```python
from build123d import *

# Parameters (mm, degrees)
SKETCH2_R           = 37.5
BOSS_EXTRUDE1_DEPTH = 6.75
SKETCH3_R           = 7.95
BOSS_EXTRUDE2_DEPTH = 150
BOSS_EXTRUDE3_DEPTH = 27


with BuildPart() as part:
    # Sketch2 → Boss-Extrude1 (new body, symmetric)
    with BuildSketch(Plane(origin=(0, 0, 0), x_dir=(1, 0, 0), z_dir=(0, 1, 0))):
        Polygon((-107, -100), (-40, -160), (40, -160), (107, -100), (107, 100), (-107, 100), align=None)
        Circle(SKETCH2_R, mode=Mode.SUBTRACT)
    extrude(amount=BOSS_EXTRUDE1_DEPTH, both=True)

    # Sketch3 → Boss-Extrude2 (add)
    with BuildSketch(Plane.XZ.offset(6.75)):
        with Locations((26.625, 147.55)):
            Circle(SKETCH3_R)
        with Locations((-26.625, 147.55)):
            Circle(SKETCH3_R)
    extrude(amount=BOSS_EXTRUDE2_DEPTH)

    # Sketch4 → Boss-Extrude3 (add)
    with BuildSketch(Plane.XZ.offset(156.75)):
        with BuildLine():
            Line((-45, 72), (-45, 160))
            Line((-45, 160), (45, 160))
            Line((45, 160), (45, 72))
            ThreePointArc((45, 72), (0, 87), (-45, 72))
        make_face()
    extrude(amount=BOSS_EXTRUDE3_DEPTH)


solid = part.part
```
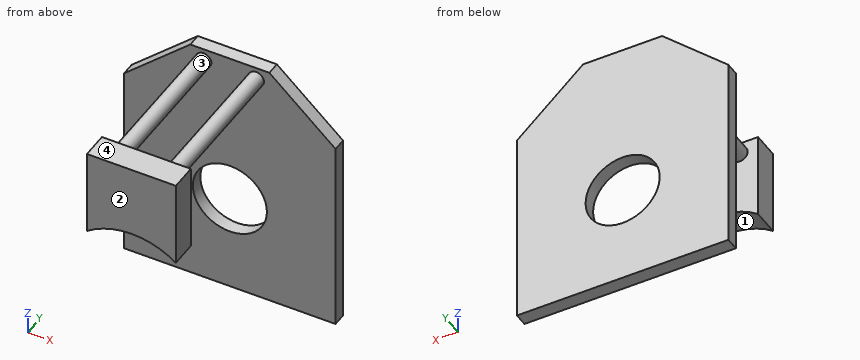
Can you work these out from the model? Positions are in its coordinate system, mm. Face numbers are marked on the shaded views. A direction names the side the tool comes from. Coordinates: 2 decimals unless noted, no trailing zeros. Order: outer loops, then holes, each group sorted by start corner. A loop starts at its lowest first (then second) coordinate and runs counter-clockwise, first axis right, second up.
1. I'm going to push flat-ended pins straight in: pin 1 (13.5 mm diameter, centred on y = -167.5, z = 106.5, fed in from +X); pin 2 (13.5 mm diameter, centred on y = -175, z = 110, fed in from -X). Where does each tip first touch, or does it pass through?
2. I need wall thicknesses on line 1 (X direction, y = 3.25, z = 0); line 2 (Z direction, x = 0, y = -1.5); line 3 (Y direction, x = 30, z = 97.5). Which ranges of each line are inside material? Lowest first, please.
3. For the marked faces 3 and 4, which set-ups out of +Z, -Z, +X, -X, +Y, -Y let a thin tool reach every point of the face, with its end or its side?
4. If we section it at C-C (y = -138): Please give me the cut outline in (x, z) (3 decimals).
5. Thinking about a two-plate mould opening in X: for the marked faces 1 and 2, which applies, +X half, -X half, draft (parallel to the pull), parting line (faces both ways), or undercut?
6. If we section it at B-B (x = 0): Please give me the cut outline in (y, z).
7. If we section it at A-A (z = 0): Please give me the cut outline in (x, y).
8. If we section it at D-D (x = -22): Please give me the cut outline in (y, z).
Entries:
1. pin 1: stops at x = 45
1. pin 2: stops at x = -45
2. line 1: x = -107 to -37.5, 37.5 to 107
2. line 2: z = -100 to -37.5, 37.5 to 160
2. line 3: y = -183.75 to -156.75, -6.75 to 6.75
3. face 3: none
3. face 4: +Z, +X, -X, +Y, -Y
4. outline: circle Ø15.9 at (-26.625, 147.55); circle Ø15.9 at (26.625, 147.55)
5. face 1: undercut
5. face 2: draft
6. outline: (-183.75, 87) - (-156.75, 87) - (-156.75, 160) - (-183.75, 160) - close; (-6.75, -100) - (6.75, -100) - (6.75, -37.5) - (-6.75, -37.5) - close; (-6.75, 37.5) - (6.75, 37.5) - (6.75, 160) - (-6.75, 160) - close
7. outline: (-107, -6.75) - (-37.5, -6.75) - (-37.5, 6.75) - (-107, 6.75) - close; (37.5, -6.75) - (107, -6.75) - (107, 6.75) - (37.5, 6.75) - close
8. outline: (-183.75, 83.7) - (-156.75, 83.7) - (-156.75, 141.08) - (-6.75, 141.08) - (-6.75, 30.37) - (6.75, 30.37) - (6.75, 160) - (-6.75, 160) - (-6.75, 154.02) - (-156.75, 154.02) - (-156.75, 160) - (-183.75, 160) - close; (-6.75, -100) - (6.75, -100) - (6.75, -30.37) - (-6.75, -30.37) - close
